Could you check a few things on this model? Use its own coordinates, in mm. A direction names the side the tool comes from. Give positions to 0.01 mm unless a question says otherwise; leave off trailing zeros. Loops run counter-clockwise (first coordinate to the right, second up) from the corner with the lowest first, then second, coordinate; pieces in that order, holes last. Notation, with made-up numbers: (64.25, 41) -> (78.25, 41) arc R27 cw to (78.25, 64) -> close; hole circle Ø1 at (68.25, -37). An arc over 180 degrees is marked (long way). Put each result on its own line as item: value.
```python
from build123d import *

# Parameters (mm, degrees)
SKETCH1_W                     = 25
SKETCH1_H                     = 15
BOSS_EXTRUDE1_DEPTH           = 1.3
BOSS_EXTRUDE2_DEPTH           = 0.1
SKETCH3_W                     = 4.723765288
SKETCH3_H                     = 5
SKETCH3_W_2                   = 2.5
SKETCH3_H_2                   = 4.03488285
BOSS_EXTRUDE3_DEPTH           = 1
SKETCH4_R                     = 0.75
BOSS_EXTRUDE4_DEPTH           = 1
BOSS_EXTRUDE4_DRAFT           = 18
BOSS_EXTRUDE4_PROFILE_2_DEPTH = 1
BOSS_EXTRUDE4_PROFILE_2_DRAFT = 18
BOSS_EXTRUDE4_PROFILE_3_DEPTH = 1
BOSS_EXTRUDE4_PROFILE_3_DRAFT = 18
BOSS_EXTRUDE4_PROFILE_4_DEPTH = 1
BOSS_EXTRUDE4_PROFILE_4_DRAFT = 18
BOSS_EXTRUDE4_PROFILE_5_DEPTH = 1
BOSS_EXTRUDE4_PROFILE_5_DRAFT = 18
BOSS_EXTRUDE4_PROFILE_6_DEPTH = 1
BOSS_EXTRUDE4_PROFILE_6_DRAFT = 18
BOSS_EXTRUDE4_PROFILE_7_DEPTH = 1
BOSS_EXTRUDE4_PROFILE_7_DRAFT = 18
BOSS_EXTRUDE4_PROFILE_8_DEPTH = 1
BOSS_EXTRUDE4_PROFILE_8_DRAFT = 18


with BuildPart() as part:
    # Sketch1 → Boss-Extrude1 (new body)
    with BuildSketch(Plane(origin=(0, 0, 0), x_dir=(1, 0, 0), z_dir=(0, 1, 0))):
        Rectangle(SKETCH1_W, SKETCH1_H)
    extrude(amount=BOSS_EXTRUDE1_DEPTH)

    # Sketch2 → Boss-Extrude2 (add)
    with BuildSketch(Plane(origin=(0, 1.3, 0), x_dir=(1, 0, 0), z_dir=(0, 1, 0))):
        Polygon((-3.654721125, -5.569339468), (-12.030839718, -5.569339468), (-12.030839718, -3.469339468), (-7.030839718, -3.469339468), (-7.030839718, -2.769339468), (-12.071748872, -2.769339468), (-12.071748872, -0.669339468), (-7.060469733, -0.669339468), (-7.060469733, 0.030660532), (-12.030839718, 0.030660532), (-12.030839718, 2.130660532), (-7.030839718, 2.130660532), (-7.030839718, 2.830660532), (-12.030839718, 2.830660532), (-12.030839718, 6.830660532), (-11.330839718, 6.830660532), (-11.330839718, 3.530660532), (-6.330839718, 3.530660532), (-6.330839718, 1.430660532), (-11.330839718, 1.430660532), (-11.330839718, 0.730660532), (-6.360469733, 0.730660532), (-6.360469733, -1.369339468), (-11.360469733, -1.369339468), (-11.360469733, -2.069339468), (-6.330839718, -2.069339468), (-6.330839718, -4.169339468), (-11.330839718, -4.169339468), (-11.330839718, -4.869339468), (-4.354721125, -4.869339468), (-4.354721125, 2.346150012), (-3.654721125, 2.346150012), align=None)
    extrude(amount=BOSS_EXTRUDE2_DEPTH)

    # Sketch3 → Boss-Extrude3 (add)
    with BuildSketch(Plane(origin=(0, 1.3, 0), x_dir=(1, 0, 0), z_dir=(0, 1, 0))):
        with Locations((0.147617665, 1.651198425)):
            Rectangle(SKETCH3_W, SKETCH3_H)
        with Locations((1.259500309, -3.727346048)):
            Rectangle(SKETCH3_W_2, SKETCH3_H_2)
    extrude(amount=BOSS_EXTRUDE3_DEPTH)


with BuildPart() as boss_extrude4_tool:
    # Sketch4 → Boss-Extrude4 (with draft: the straight prism first)
    with BuildSketch(Plane(origin=(0, 1.3, 0), x_dir=(1, 0, 0), z_dir=(0, 1, 0))):
        with Locations((7.608740396, 4.631238018)):
            Circle(SKETCH4_R)
    extrude(amount=BOSS_EXTRUDE4_DEPTH)
    # Boss-Extrude4: the draft: its side faces are tilted about the plane it starts from
    boss_extrude4_sides = [boss_extrude4_tool.faces().sort_by_distance(p)[0] for p in [
        (6.858740396, 1.8, -4.631238018),
    ]]
    draft(boss_extrude4_sides, Plane(origin=(0, 1.3, 0), x_dir=(1, 0, 0), z_dir=(0, 1, 0)), BOSS_EXTRUDE4_DRAFT)


with BuildPart() as part_1:
    add(part.part)

    # Boss-Extrude4: add boss_extrude4_tool
    add(boss_extrude4_tool.part)


with BuildPart() as boss_extrude4_profile_2_tool:
    # Sketch4 → Boss-Extrude4 profile 2 (with draft: the straight prism first)
    with BuildSketch(Plane(origin=(0, 1.3, 0), x_dir=(1, 0, 0), z_dir=(0, 1, 0))):
        with Locations((10.517617168, 4.631238018)):
            Circle(SKETCH4_R)
    extrude(amount=BOSS_EXTRUDE4_PROFILE_2_DEPTH)
    # Boss-Extrude4 profile 2: the draft: its side faces are tilted about the plane it starts from
    boss_extrude4_profile_2_sides = [boss_extrude4_profile_2_tool.faces().sort_by_distance(p)[0] for p in [
        (9.767617168, 1.8, -4.631238018),
    ]]
    draft(boss_extrude4_profile_2_sides, Plane(origin=(0, 1.3, 0), x_dir=(1, 0, 0), z_dir=(0, 1, 0)), BOSS_EXTRUDE4_PROFILE_2_DRAFT)


with BuildPart() as part_2:
    add(part_1.part)

    # Boss-Extrude4 profile 2: add boss_extrude4_profile_2_tool
    add(boss_extrude4_profile_2_tool.part)


with BuildPart() as boss_extrude4_profile_3_tool:
    # Sketch4 → Boss-Extrude4 profile 3 (with draft: the straight prism first)
    with BuildSketch(Plane(origin=(0, 1.3, 0), x_dir=(1, 0, 0), z_dir=(0, 1, 0))):
        with Locations((7.608740396, 1.631238018)):
            Circle(SKETCH4_R)
    extrude(amount=BOSS_EXTRUDE4_PROFILE_3_DEPTH)
    # Boss-Extrude4 profile 3: the draft: its side faces are tilted about the plane it starts from
    boss_extrude4_profile_3_sides = [boss_extrude4_profile_3_tool.faces().sort_by_distance(p)[0] for p in [
        (6.858740396, 1.8, -1.631238018),
    ]]
    draft(boss_extrude4_profile_3_sides, Plane(origin=(0, 1.3, 0), x_dir=(1, 0, 0), z_dir=(0, 1, 0)), BOSS_EXTRUDE4_PROFILE_3_DRAFT)


with BuildPart() as part_3:
    add(part_2.part)

    # Boss-Extrude4 profile 3: add boss_extrude4_profile_3_tool
    add(boss_extrude4_profile_3_tool.part)


with BuildPart() as boss_extrude4_profile_4_tool:
    # Sketch4 → Boss-Extrude4 profile 4 (with draft: the straight prism first)
    with BuildSketch(Plane(origin=(0, 1.3, 0), x_dir=(1, 0, 0), z_dir=(0, 1, 0))):
        with Locations((10.517617168, 1.631238018)):
            Circle(SKETCH4_R)
    extrude(amount=BOSS_EXTRUDE4_PROFILE_4_DEPTH)
    # Boss-Extrude4 profile 4: the draft: its side faces are tilted about the plane it starts from
    boss_extrude4_profile_4_sides = [boss_extrude4_profile_4_tool.faces().sort_by_distance(p)[0] for p in [
        (9.767617168, 1.8, -1.631238018),
    ]]
    draft(boss_extrude4_profile_4_sides, Plane(origin=(0, 1.3, 0), x_dir=(1, 0, 0), z_dir=(0, 1, 0)), BOSS_EXTRUDE4_PROFILE_4_DRAFT)


with BuildPart() as part_4:
    add(part_3.part)

    # Boss-Extrude4 profile 4: add boss_extrude4_profile_4_tool
    add(boss_extrude4_profile_4_tool.part)


with BuildPart() as boss_extrude4_profile_5_tool:
    # Sketch4 → Boss-Extrude4 profile 5 (with draft: the straight prism first)
    with BuildSketch(Plane(origin=(0, 1.3, 0), x_dir=(1, 0, 0), z_dir=(0, 1, 0))):
        with Locations((7.608740396, -1.368761982)):
            Circle(SKETCH4_R)
    extrude(amount=BOSS_EXTRUDE4_PROFILE_5_DEPTH)
    # Boss-Extrude4 profile 5: the draft: its side faces are tilted about the plane it starts from
    boss_extrude4_profile_5_sides = [boss_extrude4_profile_5_tool.faces().sort_by_distance(p)[0] for p in [
        (6.858740396, 1.8, 1.368761982),
    ]]
    draft(boss_extrude4_profile_5_sides, Plane(origin=(0, 1.3, 0), x_dir=(1, 0, 0), z_dir=(0, 1, 0)), BOSS_EXTRUDE4_PROFILE_5_DRAFT)


with BuildPart() as part_5:
    add(part_4.part)

    # Boss-Extrude4 profile 5: add boss_extrude4_profile_5_tool
    add(boss_extrude4_profile_5_tool.part)


with BuildPart() as boss_extrude4_profile_6_tool:
    # Sketch4 → Boss-Extrude4 profile 6 (with draft: the straight prism first)
    with BuildSketch(Plane(origin=(0, 1.3, 0), x_dir=(1, 0, 0), z_dir=(0, 1, 0))):
        with Locations((10.517617168, -1.368761982)):
            Circle(SKETCH4_R)
    extrude(amount=BOSS_EXTRUDE4_PROFILE_6_DEPTH)
    # Boss-Extrude4 profile 6: the draft: its side faces are tilted about the plane it starts from
    boss_extrude4_profile_6_sides = [boss_extrude4_profile_6_tool.faces().sort_by_distance(p)[0] for p in [
        (9.767617168, 1.8, 1.368761982),
    ]]
    draft(boss_extrude4_profile_6_sides, Plane(origin=(0, 1.3, 0), x_dir=(1, 0, 0), z_dir=(0, 1, 0)), BOSS_EXTRUDE4_PROFILE_6_DRAFT)


with BuildPart() as part_6:
    add(part_5.part)

    # Boss-Extrude4 profile 6: add boss_extrude4_profile_6_tool
    add(boss_extrude4_profile_6_tool.part)


with BuildPart() as boss_extrude4_profile_7_tool:
    # Sketch4 → Boss-Extrude4 profile 7 (with draft: the straight prism first)
    with BuildSketch(Plane(origin=(0, 1.3, 0), x_dir=(1, 0, 0), z_dir=(0, 1, 0))):
        with Locations((7.608740396, -4.368761982)):
            Circle(SKETCH4_R)
    extrude(amount=BOSS_EXTRUDE4_PROFILE_7_DEPTH)
    # Boss-Extrude4 profile 7: the draft: its side faces are tilted about the plane it starts from
    boss_extrude4_profile_7_sides = [boss_extrude4_profile_7_tool.faces().sort_by_distance(p)[0] for p in [
        (6.858740396, 1.8, 4.368761982),
    ]]
    draft(boss_extrude4_profile_7_sides, Plane(origin=(0, 1.3, 0), x_dir=(1, 0, 0), z_dir=(0, 1, 0)), BOSS_EXTRUDE4_PROFILE_7_DRAFT)


with BuildPart() as part_7:
    add(part_6.part)

    # Boss-Extrude4 profile 7: add boss_extrude4_profile_7_tool
    add(boss_extrude4_profile_7_tool.part)


with BuildPart() as boss_extrude4_profile_8_tool:
    # Sketch4 → Boss-Extrude4 profile 8 (with draft: the straight prism first)
    with BuildSketch(Plane(origin=(0, 1.3, 0), x_dir=(1, 0, 0), z_dir=(0, 1, 0))):
        with Locations((10.517617168, -4.368761982)):
            Circle(SKETCH4_R)
    extrude(amount=BOSS_EXTRUDE4_PROFILE_8_DEPTH)
    # Boss-Extrude4 profile 8: the draft: its side faces are tilted about the plane it starts from
    boss_extrude4_profile_8_sides = [boss_extrude4_profile_8_tool.faces().sort_by_distance(p)[0] for p in [
        (9.767617168, 1.8, 4.368761982),
    ]]
    draft(boss_extrude4_profile_8_sides, Plane(origin=(0, 1.3, 0), x_dir=(1, 0, 0), z_dir=(0, 1, 0)), BOSS_EXTRUDE4_PROFILE_8_DRAFT)


with BuildPart() as part_8:
    add(part_7.part)

    # Boss-Extrude4 profile 8: add boss_extrude4_profile_8_tool
    add(boss_extrude4_profile_8_tool.part)


solid = part_8.part
```
1. If we section it at A-A (z = 0.25): List the corners of the cut face in (x, y) for me, then the cut area to 3 significant figures.
Recorded:
outline: (-12.5, 0) -> (12.5, 0) -> (12.5, 1.3) -> (2.51, 1.3) -> (2.51, 2.3) -> (-2.21, 2.3) -> (-2.21, 1.3) -> (-3.65, 1.3) -> (-3.65, 1.4) -> (-4.35, 1.4) -> (-4.35, 1.3) -> (-6.36, 1.3) -> (-6.36, 1.4) -> (-7.06, 1.4) -> (-7.06, 1.3) -> (-12.5, 1.3) -> close
area: 37.4 mm^2
2. If we section it at D-D (x = -1.75): List the corners of the cut face in (y, z) for me, then the cut area to 3 significant figures.
Recorded:
outline: (0, -7.5) -> (1.3, -7.5) -> (1.3, -4.15) -> (2.3, -4.15) -> (2.3, 0.85) -> (1.3, 0.85) -> (1.3, 7.5) -> (0, 7.5) -> close
area: 24.5 mm^2
3. Thinking about a two-plate mould opening in X: for faces 1 (the face through (7.6, 2.3, -4.6)), 2 (the face through (12.5, 1, 0)), 3 (the face through (-0.2, 1.3, 1.6)), which applies, pulls with the +X half, pulls with the -X half, needs draft (parallel to the pull), parting line crosses it, or undercut?
Recorded:
face 1: needs draft
face 2: pulls with the +X half
face 3: undercut
4. For faces 4 (the face through (2.51, 2, 4)), 5 (the face through (11.01, 2.02, 4.21)), which set-ups out of +Z, -Z, +X, -X, +Y, -Y let a thin tool reach every point of the face, with its end or its side?
Recorded:
face 4: +Z, -Z, +Y
face 5: +Y
5. If we section it at C-C (y = 2.05): Count the separate pieces of the cut face and the enclosed holes in it, then the cut area to 3 significant figures.
Recorded:
separate pieces: 10
enclosed holes: 0
area: 40.1 mm^2
6. If we section it at B-B (x = 1.75): List the corners of the cut face in (y, z) for me.
Recorded:
outline: (0, -7.5) -> (1.3, -7.5) -> (1.3, -4.15) -> (2.3, -4.15) -> (2.3, 0.85) -> (1.3, 0.85) -> (1.3, 1.71) -> (2.3, 1.71) -> (2.3, 5.74) -> (1.3, 5.74) -> (1.3, 7.5) -> (0, 7.5) -> close
7. I need wall thicknesses on line 1 (X direction, y = 1.8, z = -2.75); line 2 (X direction, y = 1.75, z = 4.75); line 3 (X direction, y = 1.55, z = 2.5). Which ranges of each line are inside material? Lowest first, please.
Recorded:
line 1: x = -2.21 to 2.51
line 2: x = 0.01 to 2.51, 7.14 to 8.08, 10.05 to 10.99
line 3: x = 0.01 to 2.51
